Autodesk Inventor part; units mm, degrees
ref_plane "YZ Plane" through (0, 0, 0) normal (1, 0, 0) x (0, 1, 0)
ref_plane "XZ Plane" through (0, 0, 0) normal (0, 1, 0) x (-1, 0, 0)
ref_plane "XY Plane" through (0, 0, 0) normal (0, 0, 1) x (1, 0, 0)
sketch "Sketch1" plane through (0, 0, 0) normal (0, 0, 1) x (1, 0, 0)
  circle A0 centre (0, 0) radius 10
  arc A1 (2.4, 1.8) -> (2.4, -1.8) centre (0, 0) ccw
  line L0 (-10, 0) -> (10, 0) construction
  line L1 (0, 10) -> (0, -10) construction
  circle A2 centre (0, 0) radius 6.5 construction
  circle A3 centre (-6.5, 0) radius 1.25
  circle A4 centre (0, 6.5) radius 1.25
  circle A5 centre (0, -6.5) radius 1.25
  circle A6 centre (6.5, 0) radius 1.25
  line L2 (-3, 0) -> (0, 0) construction
  line L3 (2.4, 1.8) -> (2.4, -1.8)
  arc A7 (3, 0) -> (2.4, 1.8) centre (0, 0) ccw construction
  arc A8 (2.4, -1.8) -> (3, 0) centre (0, 0) ccw construction
  dimension "d0" = 6
  dimension "d1" = 20
  dimension "d3" = 3.5
  dimension "d4" = 2.5
  dimension "d7" = 5.4
extrude "Plate1" add sketch "Sketch1" along normal blind 2.54
equation "\"d8\" = Thickness"
equation "\"BendRadius\" = Thickness"
equation "\"BendReliefWidth\" = Thickness"
equation "\"BendReliefDepth\" = 0.5 * Thickness"
equation "\"CornerReliefSize\" = 4 * Thickness"
equation "\"MinimumRemnant\" = 2 * Thickness"
equation "\"TransitionRadius\" = BendRadius"
equation "\"JacobiRadiusSize\" = BendRadius"
equation "\"GapSize\" = Thickness"
properties part number "ForearmDHub"
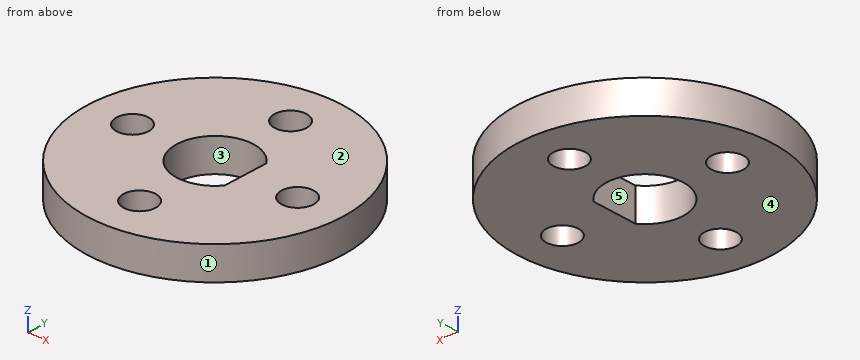
Design review of the part built by this model. Coordinates are the model's own, in mm. Face numbers are marked on the shaded views. A direction names the side the tool comes from. Round coordinates to 2 decimals unless told otherwise and drop trailing zeros. Write each loop counter-clockwise with the first axis right and the second up, starting at its lowest first coordinate (ties: lowest second). Pieces come first, ordered by that corner, then holes. Notation, with made-up numbers: M -13,-36 L 27,-36 A15 cw 27,-12 Z; hole C 87.25,-21.75 d5. An arc over 180 degrees is marked long. One line per item, written item: value. Start each with the question number.
1. Take a section at B-B on y = 0. State the section outline as (x, z) points.
2. Clearance check with flat-ended pins moving along their axes: P1, Ø1.5, axis at y = -3, z = 1, coming from the +X side; P2, Ø3, axis at x = 6.5, y = 0, coming from the +Z side; P3, Ø2, axis at x = 0, y = 6.5, coming from the +Z side. State where each tip first meets the part, or that it passes through.
3. For the marked faces 4 and 5, list the 3-axis set-ups (+Z, -Z, +X, -X, +Y, -Y) from which the entire face can be reached by the end or side of a thin tool; tool diameter is ignored.
4. Take a section at C-C on z = 1.25. State the section outline as (x, y) points, then the cut area to 3 significant figures.
5. Take a section at D-D on y = -6.5. State the section outline as (x, z) points.
6. To check wall thickness, follow probe 1 along Y at (x, z) = (0, 1.3); probe 2 along X at (y, z) = (-0.75, 2.3); probe 3 along Y at (x, z) = (0.75, 0.25). State the ranges of each line that lie inside material, in increasing order. Write a range as from..to.
7. Draft analysis for pull direction Y (two halves, no side actions). For the marked faces 1, 2 and 3, state which applies: pulls with the +Y half, pulls with the -Y half, needs draft (parallel to the pull), parting line crosses it, or undercut.
8. Take a section at A-A on x = 0. State the section outline as (y, z) points.
Computed:
1. outline: M -10,0 L -7.75,0 L -7.75,2.54 L -10,2.54 Z; M -5.25,0 L -3,0 L -3,2.54 L -5.25,2.54 Z; M 2.4,0 L 5.25,0 L 5.25,2.54 L 2.4,2.54 Z; M 7.75,0 L 10,0 L 10,2.54 L 7.75,2.54 Z
2. P1: stops at x = 9.74
2. P2: stops at z = 2.54
2. P3: passes through
3. face 4: -Z, +X, -X, +Y, -Y
3. face 5: +Z, -Z
4. outline: C 0,0 d20; hole C -6.5,0 d2.5; hole C 0,-6.5 d2.5; hole C 0,6.5 d2.5; hole M 2.4,-1.8 L 2.4,1.8 A3 ccw long Z; hole C 6.5,0 d2.5
4. area: 268 mm²
5. outline: M -7.6,0 L -1.25,0 L -1.25,2.54 L -7.6,2.54 Z; M 1.25,0 L 7.6,0 L 7.6,2.54 L 1.25,2.54 Z
6. probe 1: y = -10..-7.75, -5.25..-3, 3..5.25, 7.75..10
6. probe 2: x = -9.97..-7.5, -5.5..-2.9, 2.4..5.5, 7.5..9.97
6. probe 3: y = -9.97..-7.5, -5.5..-2.9, 2.9..5.5, 7.5..9.97
7. face 1: parting line crosses it
7. face 2: needs draft
7. face 3: undercut
8. outline: M -10,0 L -7.75,0 L -7.75,2.54 L -10,2.54 Z; M -5.25,0 L -3,0 L -3,2.54 L -5.25,2.54 Z; M 3,0 L 5.25,0 L 5.25,2.54 L 3,2.54 Z; M 7.75,0 L 10,0 L 10,2.54 L 7.75,2.54 Z
